Here's how the part is built. I have some questions about the finished solid (model axes, mm). Face numbers are marked on the shaded views. A direction names the side the tool comes from. Give positions to 0.01 mm unless a question says otherwise; leave off trailing zeros. Write each loop counter-clockwise with the first axis right and the second up, starting at its lowest first coordinate (ties: lowest second). Pieces come first, ordered by that corner, then holes. Notation, with made-up numbers: (1, 17) - (15, 17) arc R29 cw to (15, 46) - close; hole circle Ø11 at (31, 30). An arc over 180 degrees is marked (long way). Use one line per item in the form item = value. Start each with the question number.
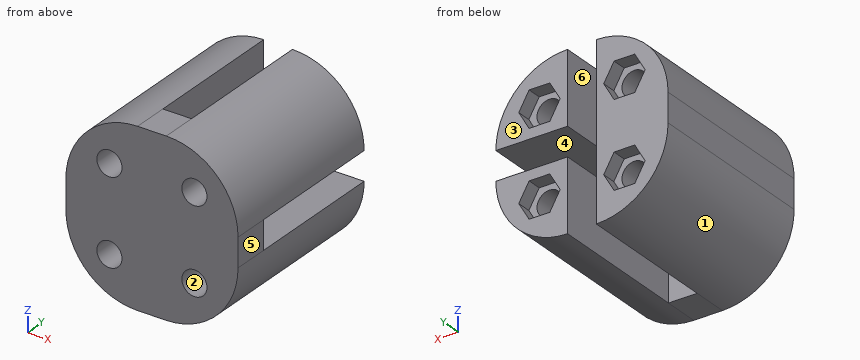
from build123d import *

# Parameters (mm, degrees)
SKETCH1_W               = 10
SKETCH1_H               = 24
BOSS_EXTRUDE1_DEPTH     = 20
BOSS_EXTRUDE1_2_DEPTH   = 20
BOSS_EXTRUDE1_3_DEPTH   = 20
BOSS_EXTRUDE2_DEPTH     = 5
FILLET1_R               = 10
SKETCH3_R               = 1.75
CUT_EXTRUDE1_DEPTH      = 29
MIRROR2_COPY_1_SKETCH_R = 1.75
MIRROR2_COPY_1_DEPTH    = 29
CUT_EXTRUDE2_DEPTH      = 2


with BuildPart() as part:
    # Sketch1 → Boss-Extrude1 (new body)
    with BuildSketch(Plane(origin=(0, 0, 0), x_dir=(1, 0, 0), z_dir=(0, 1, 0))):
        with Locations((-5, 3.136015275)):
            Rectangle(SKETCH1_W, SKETCH1_H)
    extrude(amount=BOSS_EXTRUDE1_DEPTH)



with BuildPart() as body_2:
    # Sketch1 → Boss-Extrude1 2 (new body)
    with BuildSketch(Plane(origin=(0, 0, 0), x_dir=(1, 0, 0), z_dir=(0, 1, 0))):
        with BuildLine():
            ThreePointArc((14, 1.136015275), (11.071067812, -5.935052537), (4, -8.863984725))
            Line((4, -8.863984725), (4, 1.136015275))
            Line((4, 1.136015275), (14, 1.136015275))
        make_face()
    extrude(amount=BOSS_EXTRUDE1_2_DEPTH)


with BuildPart() as body_3:
    # Sketch1 → Boss-Extrude1 3 (new body)
    with BuildSketch(Plane(origin=(0, 0, 0), x_dir=(1, 0, 0), z_dir=(0, 1, 0))):
        with BuildLine():
            ThreePointArc((4, 15.136015275), (11.071067812, 12.207083087), (14, 5.136015275))
            Line((14, 5.136015275), (4, 5.136015275))
            Line((4, 5.136015275), (4, 15.136015275))
        make_face()
    extrude(amount=BOSS_EXTRUDE1_3_DEPTH)


with BuildPart() as part_1:
    add(part.part)

    add(body_2.part)  # Boss-Extrude2 merges body 2

    add(body_3.part)  # Boss-Extrude2 merges body 3
    # Sketch2 → Boss-Extrude2 (add)
    with BuildSketch(Plane.XZ):
        with BuildLine():
            Line((-10, 8.863984725), (-10, -15.136015275))
            Line((-10, -15.136015275), (0, -15.136015275))
            Line((0, -15.136015275), (4, -15.136015275))
            ThreePointArc((4, -15.136015275), (11.071067812, -12.207083087), (14, -5.136015275))
            Line((14, -5.136015275), (14, -1.136015275))
            ThreePointArc((14, -1.136015275), (11.071067812, 5.935052537), (4, 8.863984725))
            Line((4, 8.863984725), (0, 8.863984725))
            Line((0, 8.863984725), (-10, 8.863984725))
        make_face()
    extrude(amount=BOSS_EXTRUDE2_DEPTH)

    # Fillet1
    fillet1_edges = [part_1.edges().sort_by_distance(p)[0] for p in [
        (-10, 7.5, 8.863984725),
        (-10, 7.5, -15.136015275),
    ]]
    fillet(fillet1_edges, radius=FILLET1_R - 0.0001)  # a hair under: the kernel refuses the full size

    # Sketch3 → Cut-Extrude1 (cut)
    with BuildSketch(Plane(origin=(0, 20, 0), x_dir=(1, 0, 0), z_dir=(0, 1, 0))):
        with Locations(Location((7.920878707, 9.056893982, 0), (0, 0, 270))):
            Circle(SKETCH3_R)
    cut_extrude1 = extrude(amount=-CUT_EXTRUDE1_DEPTH, mode=Mode.SUBTRACT)

    # Mirror1: Cut-Extrude1 across plane
    add(cut_extrude1.mirror(Plane.XY.offset(-3.136015275)), mode=Mode.SUBTRACT)

    # Mirror2: Cut-Extrude1 across plane
    add(cut_extrude1.mirror(Plane(origin=(2, 0, 0), x_dir=(0, 0, 1), z_dir=(1, 0, 0))), mode=Mode.SUBTRACT)

    # Mirror2 copy 1 sketch → Mirror2 copy 1 (cut)
    with BuildSketch(Plane(origin=(4, 20, -6.27203055), x_dir=(-1, 0, 0), z_dir=(0, 1, 0))):
        with Locations(Location((7.920878707, 9.056893982, 0), (0, 0, 270))):
            Circle(MIRROR2_COPY_1_SKETCH_R)
    extrude(amount=-MIRROR2_COPY_1_DEPTH, mode=Mode.SUBTRACT)

    # Sketch4 → Cut-Extrude2 (cut)
    with BuildSketch(Plane(origin=(0, 20, 0), x_dir=(1, 0, 0), z_dir=(0, 1, 0))):
        Polygon((10.807630053, 9.056893982), (9.36425438, 11.556893982), (6.477503035, 11.556893982), (5.034127362, 9.056893982), (6.477503035, 6.556893982), (9.36425438, 6.556893982), align=None)
        Polygon((10.807630053, -2.784863433), (9.36425438, -0.284863433), (6.477503035, -0.284863433), (5.034127362, -2.784863433), (6.477503035, -5.284863433), (9.36425438, -5.284863433), align=None)
        Polygon((-6.807630053, -2.784863433), (-5.36425438, -5.284863433), (-2.477503035, -5.284863433), (-1.034127362, -2.784863433), (-2.477503035, -0.284863433), (-5.36425438, -0.284863433), align=None)
        Polygon((-6.807630053, 9.056893982), (-5.36425438, 6.556893982), (-2.477503035, 6.556893982), (-1.034127362, 9.056893982), (-2.477503035, 11.556893982), (-5.36425438, 11.556893982), align=None)
    extrude(amount=-CUT_EXTRUDE2_DEPTH, mode=Mode.SUBTRACT)


solid = part_1.part
1. I want a section at B-B, the plane x = 9. List the corners of the cut face in (y, z) for me, then the cut area to 3 significant figures.
2. I want a section at D-D, the plane y = -1. List the corners of the cut face in (x, z) for me, then the cut area to 3 significant figures.
3. Please list where these lines run through material, in increasing order: line 1 (Z direction, x = -4.25, y = 14.25); line 2 (Z direction, x = -4.75, y = 18.5); line 3 (X direction, y = 8.75, z = -9).
4. I want a section at A-A, the plane y = 6. Give the number of separate pieces and of enclosed holes in the cut face, then the cut area to 3 significant figures.
5. For the marked faces 4, 5 and 6, which set-ups out of +Z, -Z, +X, -X, +Y, -Y let a thin tool reach every point of the face, with its end or its side?
6. I want a section at C-C, the plane z = -1.5. List the corners of the cut face in (x, y) for me.
7. We'd pull the mould along Z, two halves only. Please class the marked faces 1, 2 and 3: pulls with the +Z half, pulls with the -Z half, needs draft (parallel to the pull), parting line crosses it, or undercut.
8. For P1, Ø8, axis at y = 11, z = 2.5, coming from the -X side; P2, Ø1.6, axis at x = 8, y = 19, coming from the +Z side; P3, Ø1.5, axis at y = 2, z = -9, coming from the +X side; P4, Ø1, axis at x = -4.5, y = 19, coming from the -Z side, each with a flat end and sliding along its axis, tell me the tip position at first contact or that it passes through.
Result sheet:
q1.outline = (-5, -13.8) - (20, -13.8) - (20, -11.56) - (18, -11.56) - (18, -10.43) - (-5, -10.43) - close; (-5, -7.68) - (18, -7.68) - (18, -6.56) - (20, -6.56) - (20, -5.14) - (0, -5.14) - (0, -1.14) - (20, -1.14) - (20, 0.28) - (18, 0.28) - (18, 1.41) - (-5, 1.41) - close; (-5, 4.16) - (18, 4.16) - (18, 5.28) - (20, 5.28) - (20, 7.52) - (-5, 7.52) - close
q1.area = 306 mm2
q2.outline = (-10, -5.14) arc R10 ccw to (0, -15.14) - (4, -15.14) arc R10 ccw to (14, -5.14) - (14, -1.14) arc R10 ccw to (4, 8.86) - (0, 8.86) arc R10 ccw to (-10, -1.14) - close; hole circle Ø3.5 at (-3.92, -9.06); hole circle Ø3.5 at (-3.92, 2.78); hole circle Ø3.5 at (7.92, -9.06); hole circle Ø3.5 at (7.92, 2.78)
q2.area = 452 mm2
q3.line_1 = -14.19 to -10.78, -7.34 to 1.07, 4.5 to 7.92
q3.line_2 = -13.94 to -11.56, -6.56 to 0.28, 5.28 to 7.66
q3.line_3 = -9.22 to -5.67, -2.17 to 0, 4 to 6.17, 9.67 to 13.22
q4.separate_pieces = 3
q4.enclosed_holes = 4
q4.area = 316 mm2
q5.face_4 = +X, +Y
q5.face_5 = +Z, -Z, +X, +Y, -Y
q5.face_6 = +Z, -Z, +Y
q6.outline = (-10, -5) - (14, -5) - (14, 0) - (0, 0) - (0, 20) - (-10, 20) - close
q7.face_1 = pulls with the -Z half
q7.face_2 = undercut
q7.face_3 = needs draft
q8.P1 = -10
q8.P2 = 8.34
q8.P3 = 13.5
q8.P4 = -14.3
